Could you check a few things on this model? Use its own coordinates, in mm. Give positions to 0.01 mm unless a question says otherwise; leave off trailing zeros. Loops run counter-clockwise (first coordinate to the right, second up) from the corner with the lowest first, then second, coordinate; pieces in that order, holes last. Notation, with made-up numbers: M 8,63 L 65,63 A30 cw 65,88 Z; hole C 64,55.25 d7. An arc over 180 degrees is marked long. Use a Markdown table: item, result. Add a question column.
1) If I drill on line 1 along X through (y, z) = (2.6, 0); line 2 along Z through (x, y) = (-5, 1.8), over which ranges is the centre line in solid material (lowest first)? Write a range as [from, to].
2) Will this pin go through, and if not, where does the flat tip stop? pin 1 Ø8 at (x, z) = (-2.5, -5.5) entering from -Y.
3) Suppose I cut it at C-C on y = 2.7. List the corners of the cut face in (x, z) for me, and give its area (3 significant figures).
4) We'd pull the mould along Z, two halves only. Please class faces 1 (the cylindrical face through (-7.493, 1.979, -0.33)), 2 (the cylindrical face through (1.617, 2.028, 0.67)), 3 (the flat face through (1.5, 4, 1.5)): +Z half, -Z half, draft (parallel to the pull), parting line (faces both ways), or undercut.
5) Suppose I cut it at B-B on x = 0. List the corners of the cut face in (y, z) for me.
6) Suppose I cut it at A-A on z = 0. List the corners of the cut face in (x, y) for me, and give its area (3 significant figures).
```python
from build123d import *

# Parameters (mm, degrees)
SKETCH1_R           = 7.5
BOSS_EXTRUDE1_DEPTH = 4
SKETCH2_R           = 1.75
CUT_EXTRUDE1_DEPTH  = 4
FILLET1_R           = 0.5


with BuildPart() as part:
    # Sketch1 → Boss-Extrude1 (new body)
    with BuildSketch(Plane(origin=(0, 0, 0), x_dir=(1, 0, 0), z_dir=(0, 1, 0))):
        Circle(SKETCH1_R)
    extrude(amount=BOSS_EXTRUDE1_DEPTH)

    # Sketch2 → Cut-Extrude1 (cut)
    with BuildSketch(Plane(origin=(0, 4, 0), x_dir=(1, 0, 0), z_dir=(0, 1, 0))):
        Circle(SKETCH2_R)
    extrude(amount=-CUT_EXTRUDE1_DEPTH, mode=Mode.SUBTRACT)

    # Fillet1
    fillet1_edges = [part.edges().sort_by_distance(p)[0] for p in [
        (-7.5, 0, 0),
        (-7.5, 4, 0),
    ]]
    fillet(fillet1_edges, radius=FILLET1_R)


solid = part.part
```
Answer block:
| question | item | result |
|---|---|---|
| 1 | line 1 | x = [-7.5, -1.75], [1.75, 7.5] |
| 1 | line 2 | z = [-5.59, 5.59] |
| 2 | pin 1 | stops at y = 0 |
| 3 | outline | C 0,0 d15; hole C 0,0 d3.5 |
| 3 | area | 167 mm^2 |
| 4 | face 1 | parting line |
| 4 | face 2 | undercut |
| 4 | face 3 | draft |
| 5 | outline | M 0,-7 A0.5 ccw 0.5,-7.5 L 3.5,-7.5 A0.5 ccw 4,-7 L 4,-1.75 L 0,-1.75 Z; M 0,1.75 L 4,1.75 L 4,7 A0.5 ccw 3.5,7.5 L 0.5,7.5 A0.5 ccw 0,7 Z |
| 6 | outline | M -7.5,0.5 A0.5 ccw -7,0 L -1.75,0 L -1.75,4 L -7,4 A0.5 ccw -7.5,3.5 Z; M 1.75,0 L 7,0 A0.5 ccw 7.5,0.5 L 7.5,3.5 A0.5 ccw 7,4 L 1.75,4 Z |
| 6 | area | 45.8 mm^2 |
